Autodesk Inventor part; units mm, degrees
ref_plane "YZ Plane" through (0, 0, 0) normal (1, 0, 0) x (0, 1, 0)
ref_plane "XZ Plane" through (0, 0, 0) normal (0, 1, 0) x (-1, 0, 0)
ref_plane "XY Plane" through (0, 0, 0) normal (0, 0, 1) x (1, 0, 0)
sketch "Sketch1" plane through (0, 0, 0) normal (0, 0, 1) x (1, 0, 0)
  line L0 (-6.6945, 0.7224) -> (-24.6795, 0.7224)
  line L1 (-24.6795, 0.7224) -> (-24.6795, -4.2776)
  line L2 (-24.6795, -4.2776) -> (-4.6795, -4.2776)
  line L3 (-4.6795, -4.2776) -> (-4.6795, -24.2776)
  line L4 (-4.6795, -24.2776) -> (0.3205, -24.2776)
  line L5 (0.3205, -24.2776) -> (0.3205, -6.2925)
  line L6 (-6.6945, 0.7224) -> (15.2577, 22.6746)
  line L7 (22.2726, 15.6597) -> (0.3205, -6.2925)
  circle A0 centre (18.3205, 18.7224) radius 1.85
  arc A1 (22.2726, 15.6597) -> (15.2577, 22.6746) centre (18.3205, 18.7224) ccw
  dimension "d0" = 20
  dimension "d1" = 20
  dimension "d2" = 5
  dimension "d3" = 5
  dimension "d7" = 23
  dimension "d8" = 23
  dimension "d9" = 3.7
  dimension "d18" = 5
  dimension "d19" = 135
extrude "Extrusion1" add sketch "Sketch1" along normal blind 30
ref_plane "Work Plane1" through (0, 0, 24) normal (0, 0, 1) x (1, 0, 0)
sketch "Sketch3" plane through (0, 0, 24) normal (0, 0, 1) x (1, 0, 0)
  circle A0 centre (18.3205, 18.7224) radius 1.85
  circle A1 centre (18.3205, 18.7224) radius 12.5
  point P0 (0, 0)
  dimension "d13" = 25
extrude "Extrusion3" cut sketch "Sketch3" against normal blind 18
sketch "Sketch5" plane through (0, 0, 0) normal (0, 0, -1) x (-1, 0, 0)
  circle A0 centre (-18.3205, 18.7224) radius 1.85
  line L0 (24.6795, -4.2776) -> (24.6795, 0.7224)
  line L1 (24.6795, 0.7224) -> (6.6945, 0.7224)
  line L2 (6.6945, 0.7224) -> (-15.2577, 22.6746)
  arc A1 (-15.2577, 22.6746) -> (-22.2726, 15.6597) centre (-18.3205, 18.7224) ccw
  line L3 (-22.2726, 15.6597) -> (-0.3205, -6.2925)
  line L4 (-0.3205, -6.2925) -> (-0.3205, -24.2776)
  line L5 (-0.3205, -24.2776) -> (4.6795, -24.2776)
  line L6 (4.6795, -24.2776) -> (4.6795, -4.2776)
  line L7 (4.6795, -4.2776) -> (24.6795, -4.2776)
  line L8 (-0.3205, -6.2925) -> (6.6945, 0.7224)
  point P0 (0, 0)
extrude "Extrusion5" add sketch "Sketch5" along normal blind 55 contours L7 L6 L5 L4 L8 L1 L0
sketch "Sketch8" plane through (-4.6795, -24.2776, -55) normal (-1, 0, 0) x (0, 0, 1)
  circle A0 centre (10, 10) radius 2.25
  line L0 (85, 0) -> (0, 0)
  line L1 (0, 0) -> (0, 20)
  circle A1 centre (25, 10) radius 2.25
  point P0 (55, 24.2776)
  dimension "d40" = 4.5
  dimension "d41" = 10
  dimension "d42" = 10
  dimension "d43" = 4.5
  dimension "d44" = 10
  dimension "d45" = 15
sketch "Sketch9" plane through (-24.6795, 0.7224, 30) normal (0, 1, 0) x (1, 0, 0)
  circle A0 centre (10, 75) radius 2.25
  circle A1 centre (10, 60) radius 2.25
  line L0 (0, 85) -> (17.9851, 85)
  line L1 (0, 0) -> (0, 85)
  point P0 (24.6795, 30)
  dimension "d46" = 10
  dimension "d47" = 10
  dimension "d48" = 10
  dimension "d49" = 15
  dimension "d50" = 4.5
  dimension "d51" = 4.5
extrude "Extrusion8" cut sketch "Sketch9" against normal mid plane 20
extrude "Extrusion9" cut sketch "Sketch8" against normal blind 20
sketch "Sketch10" plane through (0, 0, 30) normal (0, 0, 1) x (1, 0, 0)
  line L0 (-3.9108, 3.9108) -> (4.5333, -4.5333)
  line L1 (4.5333, -4.5333) -> (4.5333, -31.01)
  line L2 (4.5333, -31.01) -> (-28.169, -31.01)
  line L3 (-28.169, -31.01) -> (-28.169, 3.9108)
  line L4 (-28.169, 3.9108) -> (-3.9108, 3.9108)
  point P0 (0, 0)
  dimension "d56" = 135
  dimension "d57" = 0
extrude "Extrusion10" cut sketch "Sketch10" against normal blind 43
sketch "Sketch11" plane through (0, 0, 0) normal (0, 0, -1) x (-1, 0, 0)
  line L0 (6.6945, 0.7224) -> (-0.3205, -6.2925)
  line L1 (-0.3205, -6.2925) -> (-17.9981, 11.3852)
  line L2 (-17.9981, 11.3852) -> (-10.9832, 18.4001)
  line L3 (-15.2577, 22.6746) -> (-6.6999, 14.1167)
  line L4 (6.6945, 0.7224) -> (-10.9832, 18.4001)
  line L5 (6.6945, 0.7224) -> (-0.3205, -6.2925)
  point P0 (0, 0)
  dimension "d60" = 25
extrude "Extrusion11" add sketch "Sketch11" along normal blind 55
equation "\"d8\" = d7"
equation "\"d43\" = d40"
equation "\"d44\" = d41"
equation "\"RodDiameter\" = 8"
equation "\"VerticalBearingOD\" = 16"
equation "\"PrintingClearance\" = 0.2"
equation "\"TubeID\" = 18"
properties part number "PulleyHolderXY"
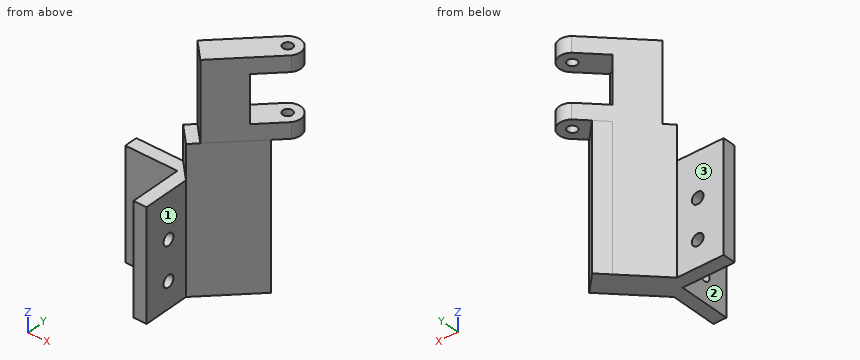
Could you check a few things on this model? Use its own coordinates, in mm. Face numbers are marked on the shaded views. A direction names the side the tool comes from. Round coordinates to 2 decimals unless told otherwise and drop trailing zeros. Loops run counter-clockwise (first coordinate to the right, second up) from the corner with the lowest first, then second, coordinate; pieces in that order, holes last. Notation, with made-up numbers: M -10,64 L 43,64 A8 ccw 43,68 Z; hole C -10.75,-39.5 d11. An arc over 180 degrees is marked long. Write item = value, one per line.
1. I want a section at D-D, the plane z = -24. Write out the boundary of the cut face in (x, y).
Results below:
outline = M -24.68,-4.28 L -4.68,-4.28 L -4.68,-24.28 L 0.32,-24.28 L 0.32,-6.29 L 18,11.39 L 10.98,18.4 L 6.7,14.12 L -6.69,0.72 L -24.68,0.72 Z
2. I want a section at A-A, the plane z = -45. Write out the boundary of the cut face in (x, y), and give its area (3 significant figures).
Results below:
outline = M -24.68,-4.28 L -16.93,-4.28 L -16.93,0.72 L -24.68,0.72 Z; M -12.43,-4.28 L -4.68,-4.28 L -4.68,-12.03 L 0.32,-12.03 L 0.32,-6.29 L 18,11.39 L 10.98,18.4 L 6.7,14.12 L -6.69,0.72 L -12.43,0.72 Z; M -4.68,-24.28 L 0.32,-24.28 L 0.32,-16.53 L -4.68,-16.53 Z
area = 403 mm²
3. Which directions (+Z, -Z, +X, -X, +Y, -Y) give clear straight access to the entire face, cutting with the end or side of a thin tool? Please do the marked faces 1, 2 and 3.
Results below:
face_1 = +Z, -Z, +X, -Y
face_2 = +Z, -Z, -X, -Y
face_3 = +Z, -Z, -X, +Y
4. Will these pins go through, and if not, where does the flat tip stop? P1, Ø5, axis at x = -7, y = -1.5, coming from the +Z side; P2, Ø3, axis at y = 12.5, z = 0, coming from the +X side; P3, Ø4, axis at y = -14.28, z = -45, coming from the -X side; P4, Ø20, axis at x = -12.5, y = -13.5, coming from the +Z side.
Results below:
P1 = 0
P2 = 20.61
P3 = through
P4 = -13
5. I want a section at C-C, the plane z = 2.5. Write out the boundary of the cut face in (x, y).
Results below:
outline = M -3.71,3.71 L 3.31,-3.31 L 22.27,15.66 A5 ccw 15.26,22.67 Z; hole C 18.32,18.72 d3.7
6. I need wall thicknesses on probe 1 along Z at (x, y) = (12.5, 12.5); probe 2 along Y at (x, z) = (-0.9, -45); probe 3 along Z at (x, y) = (-17.5, -2). Which ranges of each line are inside material? Lowest first, please.
Results below:
probe_1 = -55 to 6, 24 to 30
probe_2 = -24.28 to -16.53, -12.03 to 6.52
probe_3 = -55 to -13
